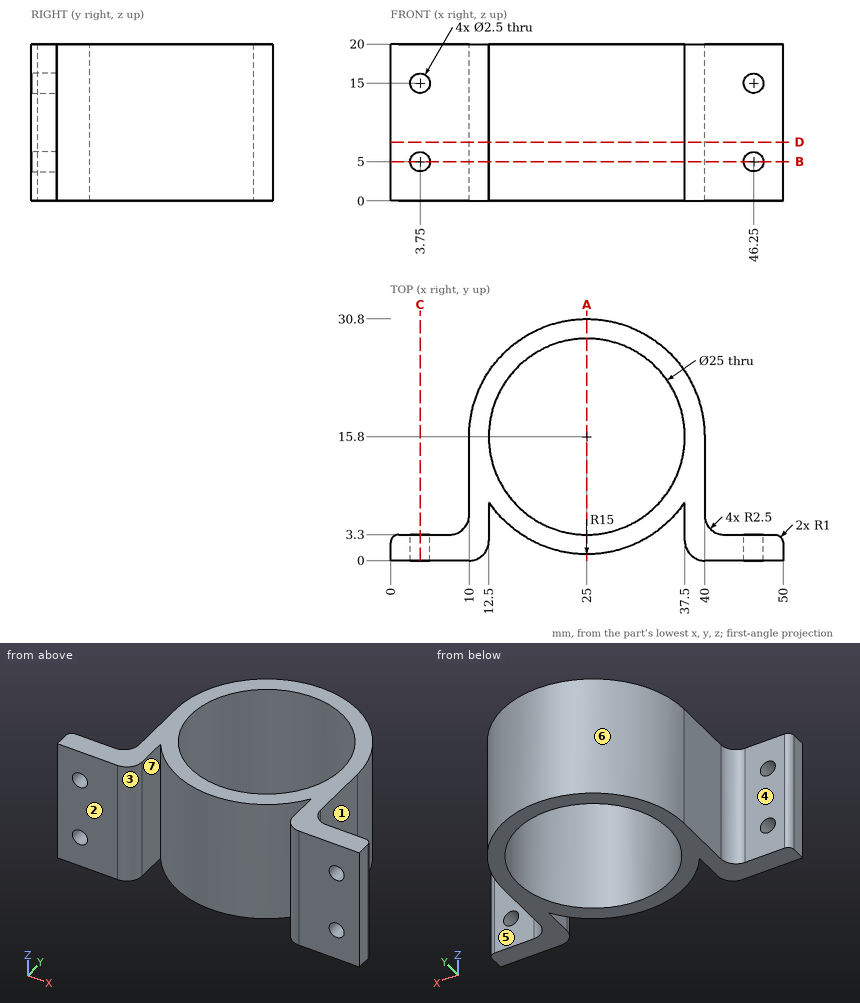
For this review, use the dimensioned drawing (mm, ordinates from the lowest corner) and the shaded views. A direction names the side the tool comes from. Round coordinates to 2 decimals unless told otherwise and drop trailing zeros. Order: outer loops, then holes, each group sorted by start corner. A loop starts at its lowest first (then second) coordinate and runs counter-clockwise, first axis right, second up. Notation, with made-up numbers: M 38,2.5 L 60,2.5 A14 ccw 60,27.5 Z; hole C 44.5,49 d10. An arc over 180 degrees is marked long. Use a Markdown table: item, result. Add a question column.
Item 1: Insertion check: pin 1 (7 mm diameter, centred on x = 45, z = 8.5, fed in from +Y); pin 2 (5 mm diameter, centred on x = 3.5, z = 9, fed in from +Y); pin 3 (3 mm diameter, centred on y = 8.5, z = 13, fed in from +X). Each pin has a flat end and moves straight along its axis. Give the tip position at first contact, or say it passes through.
Item 2: Add section C-C, the plane x = 3.75. Give the boundary of the cut face in (y, z), then the cut area to 3 significant figures.
Item 3: Tool access review of the marked faces 1, 2, 3 and 4: name each direction out of +Z, -Z, +X, -X, +Y, -Y from which nothing blocks a thin tool from reaching the whole face with its end or side.
Item 4: Add section A-A, the plane x = 25. Give the boundary of the cut face in (y, z).
Item 5: Add section B-B, the plane z = 5. Give the boundary of the cut face in (x, y).
Item 6: Mouldability with a two-part tool opening along X and no side actions: class the marked faces 5, 6 and 7 as released by +X, released by -X, zero draft, split by the parting line, or undercut.
Item 7: Add section D-D, the plane z = 7.5. Give the boundary of the cut face in (x, y), then the cut area to 3 significant figures.
Item 8: To check wall thickness, follow line 1 along Z through (x, y) = (46.25, 1.7); line 2 along Y through (x, z) = (25, 18.25); line 3 along Z through (x, y) = (3, 2). State the ranges of each line that lie inside material, in increasing order.
Geometry results:
| question | item | result |
|---|---|---|
| 1 | pin 1 | stops at y = 3.51 |
| 1 | pin 2 | stops at y = 3.3 |
| 1 | pin 3 | stops at x = 40 |
| 2 | outline | M 0,0 L 3.3,0 L 3.3,3.75 L 0,3.75 Z; M 0,6.25 L 3.3,6.25 L 3.3,13.75 L 0,13.75 Z; M 0,16.25 L 3.3,16.25 L 3.3,20 L 0,20 Z |
| 2 | area | 49.5 mm² |
| 3 | face 1 | +Z, -Z, +X, +Y |
| 3 | face 2 | +Z, -Z, +X, -X, -Y |
| 3 | face 3 | +Z, -Z, -Y |
| 3 | face 4 | +Z, -Z, -X, +Y |
| 4 | outline | M 0.8,0 L 3.3,0 L 3.3,20 L 0.8,20 Z; M 28.3,0 L 30.8,0 L 30.8,20 L 28.3,20 Z |
| 5 | outline | M 0,0 L 2.5,0 L 2.5,3.3 L 1,3.3 A1 ccw 0,2.3 Z; M 5,0 L 10,0 A2.5 ccw 12.5,2.5 L 12.5,7.51 A15 ccw 37.5,7.51 L 37.5,2.5 A2.5 ccw 40,0 L 45,0 L 45,3.3 L 42.5,3.3 A2.5 cw 40,5.8 L 40,15.8 A15 ccw 10,15.8 L 10,5.8 A2.5 cw 7.5,3.3 L 5,3.3 Z; M 47.5,0 L 50,0 L 50,2.3 A1 ccw 49,3.3 L 47.5,3.3 Z; hole C 25,15.8 d25 |
| 6 | face 5 | zero draft |
| 6 | face 6 | split by the parting line |
| 6 | face 7 | undercut |
| 7 | outline | M 0,0 L 10,0 A2.5 ccw 12.5,2.5 L 12.5,7.51 A15 ccw 37.5,7.51 L 37.5,2.5 A2.5 ccw 40,0 L 50,0 L 50,2.3 A1 ccw 49,3.3 L 42.5,3.3 A2.5 cw 40,5.8 L 40,15.8 A15 ccw 10,15.8 L 10,5.8 A2.5 cw 7.5,3.3 L 1,3.3 A1 ccw 0,2.3 Z; hole C 25,15.8 d25 |
| 7 | area | 332 mm² |
| 8 | line 1 | z = 0 to 3.75, 6.25 to 13.75, 16.25 to 20 |
| 8 | line 2 | y = 0.8 to 3.3, 28.3 to 30.8 |
| 8 | line 3 | z = 0 to 4, 6 to 14, 16 to 20 |
